from build123d import *

# Parameters (mm, degrees)
F0_W     = 180
F0_H     = 200
F0_W_2   = 177.6
F0_H_2   = 197.6
F1_DEPTH = 128
F3_DEPTH = 200.001
F5_DEPTH = 180.001


with BuildPart() as f1:
    # F0 (on Top) → F1 (new body)
    with BuildSketch(Plane.XY):
        with Locations((90, 100)):
            Rectangle(F0_W, F0_H)
        with Locations((90, 100)):
            Rectangle(F0_W_2, F0_H_2, mode=Mode.SUBTRACT)
    extrude(amount=F1_DEPTH)

    # F2 (on face) → F3 (cut, through all)
    with BuildSketch(Plane.XZ):
        Polygon((3, 121.5662565704), (3, 65.5), (84.1574190597, 65.5), align=None)
        Polygon((5.3721446832, 125), (88.5, 67.5725002305), (88.5, 125), align=None)
        Polygon((91.5, 125), (91.5, 67.5725002305), (174.6278553168, 125), align=None)
        Polygon((177, 121.5662565704), (95.8425809403, 65.5), (177, 65.5), align=None)
        Polygon((177, 62.5), (95.8425809403, 62.5), (177, 6.4337434296), align=None)
        Polygon((91.5, 60.4274997695), (91.5, 3), (174.6278553168, 3), align=None)
        Polygon((88.5, 60.4274997695), (5.3721446832, 3), (88.5, 3), align=None)
        Polygon((3, 62.5), (3, 6.4337434296), (84.1574190597, 62.5), align=None)
    extrude(amount=-F3_DEPTH, mode=Mode.SUBTRACT)

    # F4 (on face) → F5 (cut, through all)
    with BuildSketch(Plane.YZ.offset(180)):
        Polygon((3, 121.4871826042), (3, 65.5), (93.6430126453, 65.5), align=None)
        Polygon((5.1697507977, 125), (98.5, 67.3530005007), (98.5, 125), align=None)
        Polygon((101.5, 125), (101.5, 67.3530005007), (194.8302492023, 125), align=None)
        Polygon((197, 121.4871826042), (106.3569873547, 65.5), (197, 65.5), align=None)
        Polygon((197, 62.5), (106.3569873547, 62.5), (197, 6.5128173958), align=None)
        Polygon((101.5, 60.6469994993), (101.5, 3), (194.8302492023, 3), align=None)
        Polygon((98.5, 60.6469994993), (5.1697507977, 3), (98.5, 3), align=None)
        Polygon((3, 62.5), (3, 6.5128173958), (93.6430126453, 62.5), align=None)
    extrude(amount=-F5_DEPTH, mode=Mode.SUBTRACT)


solid = f1.part
Can you work these out from the model? Positions are in its coordinate system, mm. A direction names the side the tool comes from. Give positions to 0.01 mm unless a question says otherwise; leave off trailing zeros. One line per question, with ' | ' between items.
Item 1: I'm going to push a flat-ended pin straight in: pin 1 Ø12 at (x, z) = (130, 24) entering from -Y. Where does the tip first touch, or does it pass through?
Answer block:
pin 1: passes through
Item 2: Suppose I cut it at A-A, the plane y = 151. Give the number of separate pieces and of enclosed holes in the cut face, then the cut area to 3 significant figures.
Answer block:
separate pieces: 10 | enclosed holes: 0 | area: 44.9 mm2
Item 3: Please list where this line runs through material, in increasing order: L1, parallel to Y at x = 148, z = 106.
Answer block:
L1: y = 0 to 1.2, 198.8 to 200
Item 4: For faces 4 (the face through (0.61, 48.96, 93.1)), 5 (the face through (178.8, 100, 64)), 6 (the face through (44.15, 199.39, 93.14)), which set-ups out of +Z, -Z, +X, -X, +Y, -Y let a thin tool reach every point of the face, with its end or its side?
Answer block:
face 4: +X, -X | face 5: +Z, -Z | face 6: +Y, -Y
Item 5: We'd pull the mould along Y, two halves only. Please class faces 1 (the face through (89, 0, 63)), 2 (the face through (0.61, 148.82, 31.42)), 3 (the face through (0, 99, 63)): released by +Y, released by -Y, zero draft, split by the parting line, or undercut.
Answer block:
face 1: released by -Y | face 2: undercut | face 3: zero draft
